For this review, take the finished solid that the model builds, in its own axes (mm). A direction names the side the tool comes from. Give positions to 0.01 mm unless a question says otherwise; leave off trailing zeros. Order: outer loops, then holes, each group sorted by start corner. A loop starts at its lowest first (then second) coordinate and runs counter-clockwise, first axis right, second up. Notation, with made-up numbers: (15, 13.25) -> (74, 13.25) arc R24 ccw to (74, 33.25) -> close; hole circle Ø4 at (64, -20.75). An arc over 180 degrees is marked (long way). One line per item, written item: value. Start each with the question number.
from build123d import *

# Parameters (mm, degrees)
F0_R     = 3.175
F1_DEPTH = 12.7
F2_DEPTH = 25.4


with BuildPart() as f1:
    # F0 (on Front) → F1 (new body, symmetric)
    with BuildSketch(Plane.XZ):
        with BuildLine():
            ThreePointArc((-9.2225415932, 78.58125), (-1.2001908859, 66.7509171431), (9.525, 76.2))
            ThreePointArc((9.525, 76.2), (9.4490828569, 77.4001908859), (9.2225415932, 78.58125))
            ThreePointArc((9.2225415932, 78.58125), (0, 85.725), (-9.2225415932, 78.58125))
        make_face()
        with Locations((0, 76.2)):
            Circle(F0_R, mode=Mode.SUBTRACT)
        with BuildLine():
            ThreePointArc((9.2225415932, 78.58125), (9.4490828569, 77.4001908859), (9.525, 76.2))
            ThreePointArc((9.525, 76.2), (-1.2001908859, 66.7509171431), (-9.2225415932, 78.58125))
            Line((-9.2225415932, 78.58125), (-21.5192637174, 30.95625))
            ThreePointArc((-21.5192637174, 30.95625), (0, 47.625), (21.5192637174, 30.95625))
            Line((21.5192637174, 30.95625), (9.2225415932, 78.58125))
        make_face()
        with Locations((-7.0844171569, 61.9252)):
            Circle(F0_R, mode=Mode.SUBTRACT)
        with BuildLine():
            ThreePointArc((22.225, 25.4), (22.0478599995, 28.2004454004), (21.5192637174, 30.95625))
            ThreePointArc((21.5192637174, 30.95625), (0, 47.625), (-21.5192637174, 30.95625))
            ThreePointArc((-21.5192637174, 30.95625), (-22.204821299, 26.3468558918), (-21.9141455299, 21.6958333333))
            ThreePointArc((-21.9141455299, 21.6958333333), (-0.0201347951, 3.1750091206), (21.9073979622, 21.6561330786))
            ThreePointArc((21.9073979622, 21.6561330786), (22.1454571494, 23.5213428613), (22.225, 25.4))
        make_face()
        with Locations((0, 25.4)):
            Circle(F0_R, mode=Mode.SUBTRACT)
        with BuildLine():
            ThreePointArc((21.9073979622, 21.6561330786), (-0.0201347951, 3.1750091206), (-21.9141455299, 21.6958333333))
            Line((-21.9141455299, 21.6958333333), (-9.3917766557, -52.3875))
            ThreePointArc((-9.3917766557, -52.3875), (-0.7965401292, -41.3083642704), (9.525, -50.8))
            ThreePointArc((9.525, -50.8), (7.0085890152, -57.2502174394), (0.7889779495, -60.2922673158))
            Line((0.7889779495, -60.2922673158), (38.4290236064, -58.730677759))
            ThreePointArc((38.4290236064, -58.730677759), (30.1625, -50.8), (38.4290236064, -42.869322241))
            Line((38.4290236064, -42.869322241), (20.1036312885, -42.1090484218))
            ThreePointArc((20.1036312885, -42.1090484218), (14.2515043463, -39.1649364905), (12.5965921187, -32.8264468968))
            Line((12.5965921187, -32.8264468968), (21.9073979622, 21.6561330786))
        make_face()
        with BuildLine():
            ThreePointArc((9.525, -50.8), (-0.7965401292, -41.3083642704), (-9.3917766557, -52.3875))
            ThreePointArc((-9.3917766557, -52.3875), (-6.1483610621, -58.0748389157), (0, -60.325))
            Line((0, -60.325), (0.7889779495, -60.2922673158))
            ThreePointArc((0.7889779495, -60.2922673158), (7.0085890152, -57.2502174394), (9.525, -50.8))
        make_face()
        with Locations((0, -50.8)):
            Circle(F0_R, mode=Mode.SUBTRACT)
        with BuildLine():
            Line((0.7889779495, -60.2922673158), (0, -60.325))
            ThreePointArc((0, -60.325), (0.3948283277, -60.3168133107), (0.7889779495, -60.2922673158))
        make_face()
        with BuildLine():
            ThreePointArc((46.0375, -50.8), (43.8278063482, -45.3048984826), (38.4290236064, -42.869322241))
            ThreePointArc((38.4290236064, -42.869322241), (30.1625, -50.8), (38.4290236064, -58.730677759))
            ThreePointArc((38.4290236064, -58.730677759), (43.8278063482, -56.2951015174), (46.0375, -50.8))
        make_face()
        with Locations((38.1, -50.8)):
            Circle(F0_R, mode=Mode.SUBTRACT)
    extrude(amount=F1_DEPTH, both=True)

    # F0 (on Front) → F2 (join)
    with BuildSketch(Plane.XZ):
        with BuildLine():
            ThreePointArc((-9.2225415932, 78.58125), (-1.2001908859, 66.7509171431), (9.525, 76.2))
            ThreePointArc((9.525, 76.2), (9.4490828569, 77.4001908859), (9.2225415932, 78.58125))
            ThreePointArc((9.2225415932, 78.58125), (0, 85.725), (-9.2225415932, 78.58125))
        make_face()
        with Locations((0, 76.2)):
            Circle(F0_R, mode=Mode.SUBTRACT)
        with BuildLine():
            ThreePointArc((9.2225415932, 78.58125), (9.4490828569, 77.4001908859), (9.525, 76.2))
            ThreePointArc((9.525, 76.2), (-1.2001908859, 66.7509171431), (-9.2225415932, 78.58125))
            Line((-9.2225415932, 78.58125), (-21.5192637174, 30.95625))
            ThreePointArc((-21.5192637174, 30.95625), (0, 47.625), (21.5192637174, 30.95625))
            Line((21.5192637174, 30.95625), (9.2225415932, 78.58125))
        make_face()
        with Locations((-7.0844171569, 61.9252)):
            Circle(F0_R, mode=Mode.SUBTRACT)
        with BuildLine():
            ThreePointArc((22.225, 25.4), (22.0478599995, 28.2004454004), (21.5192637174, 30.95625))
            ThreePointArc((21.5192637174, 30.95625), (0, 47.625), (-21.5192637174, 30.95625))
            ThreePointArc((-21.5192637174, 30.95625), (-22.204821299, 26.3468558918), (-21.9141455299, 21.6958333333))
            ThreePointArc((-21.9141455299, 21.6958333333), (-0.0201347951, 3.1750091206), (21.9073979622, 21.6561330786))
            ThreePointArc((21.9073979622, 21.6561330786), (22.1454571494, 23.5213428613), (22.225, 25.4))
        make_face()
        with Locations((0, 25.4)):
            Circle(F0_R, mode=Mode.SUBTRACT)
        with BuildLine():
            ThreePointArc((21.9073979622, 21.6561330786), (-0.0201347951, 3.1750091206), (-21.9141455299, 21.6958333333))
            Line((-21.9141455299, 21.6958333333), (-9.3917766557, -52.3875))
            ThreePointArc((-9.3917766557, -52.3875), (-0.7965401292, -41.3083642704), (9.525, -50.8))
            ThreePointArc((9.525, -50.8), (7.0085890152, -57.2502174394), (0.7889779495, -60.2922673158))
            Line((0.7889779495, -60.2922673158), (38.4290236064, -58.730677759))
            ThreePointArc((38.4290236064, -58.730677759), (30.1625, -50.8), (38.4290236064, -42.869322241))
            Line((38.4290236064, -42.869322241), (20.1036312885, -42.1090484218))
            ThreePointArc((20.1036312885, -42.1090484218), (14.2515043463, -39.1649364905), (12.5965921187, -32.8264468968))
            Line((12.5965921187, -32.8264468968), (21.9073979622, 21.6561330786))
        make_face()
        with BuildLine():
            ThreePointArc((9.525, -50.8), (-0.7965401292, -41.3083642704), (-9.3917766557, -52.3875))
            ThreePointArc((-9.3917766557, -52.3875), (-6.1483610621, -58.0748389157), (0, -60.325))
            Line((0, -60.325), (0.7889779495, -60.2922673158))
            ThreePointArc((0.7889779495, -60.2922673158), (7.0085890152, -57.2502174394), (9.525, -50.8))
        make_face()
        with Locations((0, -50.8)):
            Circle(F0_R, mode=Mode.SUBTRACT)
        with BuildLine():
            Line((0.7889779495, -60.2922673158), (0, -60.325))
            ThreePointArc((0, -60.325), (0.3948283277, -60.3168133107), (0.7889779495, -60.2922673158))
        make_face()
        with BuildLine():
            ThreePointArc((46.0375, -50.8), (43.8278063482, -45.3048984826), (38.4290236064, -42.869322241))
            ThreePointArc((38.4290236064, -42.869322241), (30.1625, -50.8), (38.4290236064, -58.730677759))
            ThreePointArc((38.4290236064, -58.730677759), (43.8278063482, -56.2951015174), (46.0375, -50.8))
        make_face()
        with Locations((38.1, -50.8)):
            Circle(F0_R, mode=Mode.SUBTRACT)
    extrude(amount=F2_DEPTH)


solid = f1.part
Q1. For pin 1 Ø5.5 at (x, z) = (0, -50.8) entering from +Y; pin 2 Ø10 at (y, z) = (-9, 62) entering from -X; pin 3 Ø12 at (y, z) = (-12, -37) entering from -X; pin 4 Ø6 at (y, z) = (0.5, -9) entering from +X, all flat-tipped, find the tip position at first contact; note any pin that passes through.
Q2. Take a section at A-A (z = 25.4). State the section outline as (x, y) points (3 decimals), and give its area (3 significant figures).
Q3. Take a section at D-D (z = -50.8). State the section outline as (x, y) points (1 decimal).
Q4. Take a section at B-B (x = -6). State the section outline as (y, z) points.
Q5. For faces 5 (the flat face through (-15.285, -6.083, 55.102)), 6 (the flat face through (17.187, -6.083, -5.967)), list the 3-axis set-ups (+Z, -Z, +X, -X, +Y, -Y) from which the entire face can be reached by the end or side of a thin tool; tool diameter is ignored.
Q6. For line 1 along Z through (x, y) = (38.1, -18) (3 decimals); line 2 along X through (y, z) = (0, 29); line 3 along X through (y, z) = (-20, 35), list the stretches that pass through material, from the lowest coordinate up.
Q7. Mouldability with a two-part tool opening along Z and no side actions: class faces 1 (the cylindrical face through (14.311, -6.083, -39.238)), 2 (the flat face through (4, 12.7, 14)), 3 (the cylindrical face through (46.036, -6.083, -50.97)), 4 (the cylindrical face through (37.69, -6.08, -47.65)) as pulls with the +Z half, pulls with the -Z half, needs draft (parallel to the pull), parting line crosses it, or undercut.
Q8. Take a section at C-C (y = -13.5). State how many separate pieces and enclosed holes the cut face has, and give its area (3 significant figures).
Answers below:
1. pin 1: passes through
1. pin 2: stops at x = -14.79
1. pin 3: stops at x = -13.01
1. pin 4: stops at x = 17.18
2. outline: (-22.225, -25.4) -> (-3.175, -25.4) -> (-3.175, 12.7) -> (-22.225, 12.7) -> close; (3.175, -25.4) -> (22.225, -25.4) -> (22.225, 12.7) -> (3.175, 12.7) -> close
2. area: 1,450 mm²
3. outline: (-9.7, -25.4) -> (-3.2, -25.4) -> (-3.2, 12.7) -> (-9.7, 12.7) -> close; (3.2, -25.4) -> (34.9, -25.4) -> (34.9, 12.7) -> (3.2, 12.7) -> close; (41.3, -25.4) -> (46, -25.4) -> (46, 12.7) -> (41.3, 12.7) -> close
4. outline: (-25.4, -58.2) -> (12.7, -58.2) -> (12.7, 58.94) -> (-25.4, 58.94) -> close; (-25.4, 64.91) -> (12.7, 64.91) -> (12.7, 83.6) -> (-25.4, 83.6) -> close
5. face 5: +Z, -X, +Y, -Y
5. face 6: +X, +Y, -Y
6. line 1: z = -58.744 to -53.975, -47.625 to -42.856
6. line 2: x = -21.93 to 21.93
6. line 3: x = -20.48 to 20.48
7. face 1: undercut
7. face 2: needs draft
7. face 3: parting line crosses it
7. face 4: undercut
8. separate pieces: 1
8. enclosed holes: 5
8. area: 4,850 mm²
